Geometry check sheet. Reference: the model listing, model coordinates, mm. A direction names the side the tool comes from. Round coordinates to 2 decimals unless told otherwise and drop trailing zeros. Write each loop counter-clockwise with the first axis right and the second up, starting at its lowest first coordinate (ties: lowest second). Pieces come first, ordered by that corner, then holes.
Item 1: Cross-section at B-B (x = 13). Enter the section's corners in (y, z), then the cut area to 3 significant figures.
Item 2: Depth check by flat-ended pin: P1, Ø12, axis at x = 10, y = 1.5, coming from the +Z side. Enter the tip coordinate at first touch or a pass-through.
Item 3: Cross-section at C-C (z = 0.7). Enter the section's corners in (x, y).
Item 4: Cross-section at D-D (y = 5.5). Enter the section's corners in (x, z).
Item 5: Draft check along Y on faces 3 (the face through (0, -14, 1)), 4 (the face through (18.9, 8, 1)), 5 (the face through (0, -12, 2)). Enter one of: pulls with the +Y half, pulls with the -Y half, needs draft (parallel to the pull), parting line crosses it, or undercut.
Item 6: Cross-section at A-A (y = 8.5). Enter the section's corners in (x, z).
Item 7: Scan lines: probe 1 along X at (y, z) = (7, 1.45); probe 2 along Y at (x, z) = (-3, 0.8); probe 3 along X at (y, z) = (-6.5, 0.5). Record each from-to range of solid material in increasing order.
Item 8: Access from +Z, -Z, +X, -X, +Y, -Y to the whole of each face (thin tool, end or side, straight path). Record for faces 1 (the face through (-27, 0, 1)), 2 (the face through (-23.1, -9, 1)).
from build123d import *

# Parameters (mm, degrees)
SKETCH_1_W                               = 54
SKETCH_1_H                               = 28
GAUGE_PLATE_2MM_DEPTH                    = 2
OPEN_WINDOW_START                        = -0.1
SKETCH_2_W                               = 34
SKETCH_2_H                               = 20
OPEN_WINDOW_DEPTH                        = 2.2
SAME_SLOTS_AS_SENSOR_BRACKET_42X17_START = -0.1
SKETCH_3_W                               = 4.2
SKETCH_3_H                               = 3.6
SAME_SLOTS_AS_SENSOR_BRACKET_42X17_DEPTH = 2.2


with BuildPart() as part:
    # 草图1 → Gauge_plate_2mm (new body)
    with BuildSketch(Plane.XY):
        Rectangle(SKETCH_1_W, SKETCH_1_H)
    extrude(amount=GAUGE_PLATE_2MM_DEPTH)

    # 草图2 → Open_window (cut)
    with BuildSketch(Plane.XY.offset(OPEN_WINDOW_START)):
        Rectangle(SKETCH_2_W, SKETCH_2_H)
    extrude(amount=OPEN_WINDOW_DEPTH, mode=Mode.SUBTRACT)

    # 草图3 → Same_slots_as_sensor_bracket_42x17 (cut)
    with BuildSketch(Plane.XY.offset(SAME_SLOTS_AS_SENSOR_BRACKET_42X17_START)):
        with Locations((-21, -8.5)):
            Rectangle(SKETCH_3_W, SKETCH_3_H)
        with Locations((-21, 8.5)):
            Rectangle(SKETCH_3_W, SKETCH_3_H)
        with Locations((21, -8.5)):
            Rectangle(SKETCH_3_W, SKETCH_3_H)
        with Locations((21, 8.5)):
            Rectangle(SKETCH_3_W, SKETCH_3_H)
    extrude(amount=SAME_SLOTS_AS_SENSOR_BRACKET_42X17_DEPTH, mode=Mode.SUBTRACT)


solid = part.part
Resolved:
1. outline: (-14, 0) - (-10, 0) - (-10, 2) - (-14, 2) - close; (10, 0) - (14, 0) - (14, 2) - (10, 2) - close
1. area: 16.0 mm2
2. P1: passes through
3. outline: (-27, -14) - (27, -14) - (27, 14) - (-27, 14) - close; hole (-23.1, -10.3) - (-18.9, -10.3) - (-18.9, -6.7) - (-23.1, -6.7) - close; hole (-23.1, 6.7) - (-18.9, 6.7) - (-18.9, 10.3) - (-23.1, 10.3) - close; hole (-17, -10) - (17, -10) - (17, 10) - (-17, 10) - close; hole (18.9, -10.3) - (23.1, -10.3) - (23.1, -6.7) - (18.9, -6.7) - close; hole (18.9, 6.7) - (23.1, 6.7) - (23.1, 10.3) - (18.9, 10.3) - close
4. outline: (-27, 0) - (-17, 0) - (-17, 2) - (-27, 2) - close; (17, 0) - (27, 0) - (27, 2) - (17, 2) - close
5. face 3: pulls with the -Y half
5. face 4: undercut
5. face 5: needs draft
6. outline: (-27, 0) - (-23.1, 0) - (-23.1, 2) - (-27, 2) - close; (-18.9, 0) - (-17, 0) - (-17, 2) - (-18.9, 2) - close; (17, 0) - (18.9, 0) - (18.9, 2) - (17, 2) - close; (23.1, 0) - (27, 0) - (27, 2) - (23.1, 2) - close
7. probe 1: x = -27 to -23.1, -18.9 to -17, 17 to 18.9, 23.1 to 27
7. probe 2: y = -14 to -10, 10 to 14
7. probe 3: x = -27 to -17, 17 to 27
8. face 1: +Z, -Z, -X, +Y, -Y
8. face 2: +Z, -Z
